```python
from build123d import *

# Parameters (mm, degrees)
F0_W     = 50
F0_H     = 50
F0_W_2   = 44
F0_H_2   = 44
F1_DEPTH = 1150
F2_R     = 2
F3_R     = 5
F5_D     = 18


with BuildPart() as f1:
    # F0 (on Top) → F1 (new body)
    with BuildSketch(Plane.XY):
        Rectangle(F0_W, F0_H)
        Rectangle(F0_W_2, F0_H_2, mode=Mode.SUBTRACT)
    extrude(amount=F1_DEPTH)

    # F2
    f2_edges = [f1.edges().sort_by_distance(p)[0] for p in [
        (22, 22, 575),
        (-22, -22, 575),
        (-22, 22, 575),
        (22, -22, 575),
    ]]
    fillet(f2_edges, radius=F2_R)

    # F3
    f3_edges = [f1.edges().sort_by_distance(p)[0] for p in [
        (-25, 25, 575),
        (25, 25, 575),
        (-25, -25, 575),
        (25, -25, 575),
    ]]
    fillet(f3_edges, radius=F3_R)

    # F5 (through all)
    with Locations(Plane.YZ.offset(25)):
        with Locations((0, 150)):
            Hole(F5_D / 2)


solid = f1.part
```
Model file for the job. Use its own axes, mm. A direction names the side the tool comes from. Round coordinates to 2 decimals unless told otherwise and drop trailing zeros. Loops run counter-clockwise (first coordinate to the right, second up) from the corner with the lowest first, then second, coordinate; pieces in that order, holes last. Notation, with made-up numbers: M 58,23.5 L 84,23.5 A9 cw 84,38.5 Z; hole C -32.5,8 d1. An arc over 180 degrees is marked long. Put each result on its own line as item: value. Start each with the question number.
Item 1: Cut at C-C (z = 424.5). List the corners of the cut face in (x, y), then the cut area to 3 significant figures.
Item 2: Cut at A-A (y = 0). List the corners of the cut face in (x, z).
Item 3: Cut at B-B (x = -7). List the corners of the cut face in (y, z).
Item 4: Drill centre lines: line 1 along Y through (x, z) = (7, 178.5); line 2 along Z through (x, y) = (24, 0). Where is each one in solid material? Low to high.
Item 5: Mould opens along Z. For faces 3 (the face through (0, -22, 567)), 4 (the face through (-23.521, 1.172, 158.923)), 5 (the face through (23.479, 1.172, 158.923)), 6 (the face through (-22.3, 2, 0)) say: released by +Z, released by -Z, zero draft, split by the parting line, or undercut.
Item 6: 3-axis set-ups, long thin cutter, end or side, ignore diameter. For faces 1 (the face through (-25, 0, 567)), 2 (the face through (0, 22, 567)): which of +Z, -Z, +X, -X, +Y, -Y reach the whole face in a straight line?
Answer block:
1. outline: M -25,-20 A5 ccw -20,-25 L 20,-25 A5 ccw 25,-20 L 25,20 A5 ccw 20,25 L -20,25 A5 ccw -25,20 Z; hole M -22,-20 A2 ccw -20,-22 L 20,-22 A2 ccw 22,-20 L 22,20 A2 ccw 20,22 L -20,22 A2 ccw -22,20 Z
1. area: 546 mm2
2. outline: M -25,0 L -22,0 L -22,141 L -25,141 Z; M -25,159 L -22,159 L -22,1150 L -25,1150 Z; M 22,0 L 25,0 L 25,141 L 22,141 Z; M 22,159 L 25,159 L 25,1150 L 22,1150 Z
3. outline: M -25,0 L -22,0 L -22,1150 L -25,1150 Z; M 22,0 L 25,0 L 25,1150 L 22,1150 Z
4. line 1: -25 to -22, 22 to 25
4. line 2: 0 to 141, 159 to 1150
5. face 3: zero draft
5. face 4: undercut
5. face 5: undercut
5. face 6: released by -Z
6. face 1: +Z, -Z, -X, +Y, -Y
6. face 2: +Z, -Z
